from build123d import *

# Parameters (mm, degrees)
F0_W     = 220
F0_H     = 220
F1_DEPTH = 2
F2_R     = 2
F3_DEPTH = 25
F4_W     = 200
F4_H     = 200
F5_DEPTH = 1


with BuildPart() as f1:
    # F0 (on Top) → F1 (new body)
    with BuildSketch(Plane.XY):
        Rectangle(F0_W, F0_H)
    extrude(amount=F1_DEPTH)

    # F2 (on face) → F3 (cut)
    with BuildSketch(Plane.XY.offset(2)):
        with Locations((-105, -105)):
            Circle(F2_R)
        with Locations((105, -105)):
            Circle(F2_R)
        with Locations((105, 105)):
            Circle(F2_R)
        with Locations((-105, 105)):
            Circle(F2_R)
    extrude(amount=-F3_DEPTH, mode=Mode.SUBTRACT)

    # F4 (on face) → F5 (join)
    with BuildSketch(Plane.XY.offset(2)):
        Rectangle(F4_W, F4_H)
    extrude(amount=F5_DEPTH)


solid = f1.part
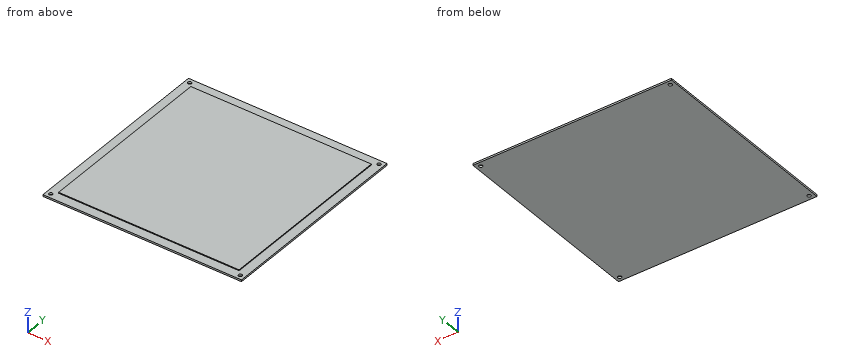
Could you check a few things on this model? Use its own coordinates, in mm. Give positions to 0.01 mm unless a question says otherwise; leave off trailing zeros. Write each loop counter-clockwise with the first axis right and the second up, starting at its lowest first coordinate (ties: lowest second). Pieces come first, ordered by that corner, then holes. Notation, with made-up numbers: (80.25, 70.5) -> (88.25, 70.5) arc R32 ccw to (88.25, 96.5) -> close; hole circle Ø10 at (85.5, -7). An arc over 180 degrees is marked (long way). Write each question's results on one line, items separated by ' | '. Start each with the question number.
Q1. Suppose I cut it at C-C, the plane z = 2.5. List the corners of the cut face in (x, y) for me.
Q2. I'm going to push flat-ended pins straight in: pin 1 Ø0.8 at (y, z) = (-9.5, 2.5) entering from +X; pin 2 Ø0.8 at (x, z) = (-49, 2.5) entering from -Y; pin 3 Ø6.5 at (x, y) = (105, 105) entering from +Z. Where does each tip first touch, or does it pass through?
Q3. Suppose I cut it at A-A, the plane x = -43.5. List the corners of the cut face in (y, z) for me.
Q4. I need wall thicknesses on probe 1 along Y at (x, z) = (-105, 0.5); probe 2 along X at (y, z) = (79, 2.1). Which ranges of each line are inside material? Lowest first, please.
Outcome:
1) outline: (-100, -100) -> (100, -100) -> (100, 100) -> (-100, 100) -> close
2) pin 1: x = 100 | pin 2: y = -100 | pin 3: z = 2
3) outline: (-110, 0) -> (110, 0) -> (110, 2) -> (100, 2) -> (100, 3) -> (-100, 3) -> (-100, 2) -> (-110, 2) -> close
4) probe 1: -110 to -107, -103 to 103, 107 to 110 | probe 2: -100 to 100
